Model file for the job. Use its own axes, mm. Face numbers are marked on the shaded views. A direction names the side the tool comes from. Round coordinates to 2 decimals unless told otherwise and drop trailing zeros. Order: outer loops, then holes, each group sorted by start corner. A loop starts at its lowest first (then second) coordinate and runs counter-clockwise, first axis right, second up. Notation, with made-up numbers: (51, -25) - (96, -25) arc R9 ccw to (96, -14) - close; hole circle Ø3 at (-3, -21.75). An arc over 180 degrees is marked (long way). Write item = value, one per line.
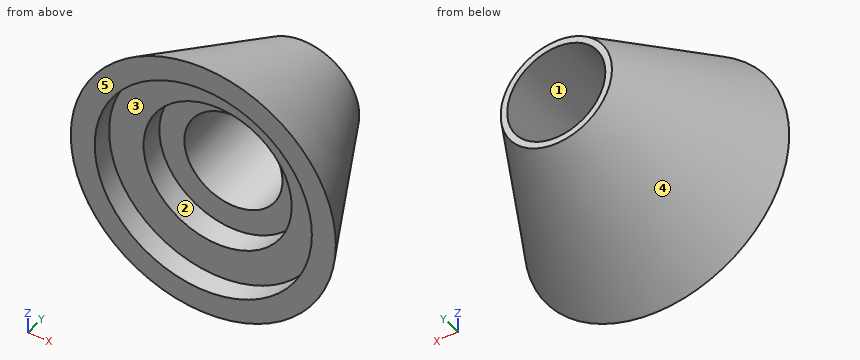
```python
from build123d import *

# Parameters (mm, degrees)
F2_R     = 4.702761
F3_DEPTH = 25.4
F5_R     = 7.100164
F6_DEPTH = 4.4196
F7_R     = 10.405199
F8_DEPTH = 2.1082


with BuildPart() as f1:
    # F0 (on Top) → F1 (revolve)
    with BuildSketch(Plane.XY):
        Polygon((0, -10.469328), (0, 4.262672), (-5.334, 4.262672), (-12.7, -10.469328), align=None)
    revolve(axis=Axis((0, 2.230672, 0), (0, -1, 0)))

    # F2 (on face) → F3 (cut)
    with BuildSketch(Plane(origin=(0, 4.262672, 0), x_dir=(-1, 0, 0), z_dir=(0, 1, 0))):
        Circle(F2_R)
    extrude(amount=-F3_DEPTH, mode=Mode.SUBTRACT)

    # F5 (on face) → F6 (cut)
    with BuildSketch(Plane.XZ.offset(10.469328)):
        Circle(F5_R)
    extrude(amount=-F6_DEPTH, mode=Mode.SUBTRACT)

    # F7 (on face) → F8 (cut)
    with BuildSketch(Plane.XZ.offset(10.469328)):
        Circle(F7_R)
    extrude(amount=-F8_DEPTH, mode=Mode.SUBTRACT)


solid = f1.part
```
1) Wall check: line 1 along X through (y, z) = (-2.75, -0.5); line 2 along Z through (x, y) = (0.75, -4); line 3 along Z through (x, y) = (0, -9.35). Give the ranges that are in metal, low to high.
Conclusion:
line_1 = -8.83 to -4.68, 4.68 to 8.83
line_2 = -9.44 to -4.64, 4.64 to 9.44
line_3 = -12.14 to -10.41, 10.41 to 12.14
2) Cut at B-B (x = 0). Write the cut outline in (y, z).
Conclusion:
outline = (-10.47, -12.7) - (4.26, -5.33) - (4.26, -4.7) - (-6.05, -4.7) - (-6.05, -7.1) - (-8.36, -7.1) - (-8.36, -10.41) - (-10.47, -10.41) - close; (-10.47, 10.41) - (-8.36, 10.41) - (-8.36, 7.1) - (-6.05, 7.1) - (-6.05, 4.7) - (4.26, 4.7) - (4.26, 5.33) - (-10.47, 12.7) - close
3) Cut at D-D (y = -1.5). Write the cut outline in (x, z), and give its area (3 significant figures).
Conclusion:
outline = circle Ø16.43 at (0, 0); hole circle Ø9.41 at (0, 0)
area = 143 mm^2
4) 3-axis set-ups, long thin cutter, end or side, ignore diameter. For the marked faces 1 and 2: which of +Z, -Z, +X, -X, +Y, -Y reach the whole face in a straight line?
Conclusion:
face_1 = +Y, -Y
face_2 = -Y
5) Mould opens along X. For the marked faces 3, 4 and 5 say: +X half, -X half, draft (parallel to the pull), parting line (faces both ways), or undercut.
Conclusion:
face_3 = undercut
face_4 = parting line
face_5 = draft
6) Cut at C-C (y = -7). Write the cut outline in (x, z), and give its area (3 significant figures).
Conclusion:
outline = circle Ø21.93 at (0, 0); hole circle Ø14.2 at (0, 0)
area = 219 mm^2
7) Flat gauge pins, fed straight in: pin 1 Ø5 at (y, z) = (1.5, -4.5) entering from +X; pin 2 Ø4 at (y, z) = (-3, -9.5) entering from -X; pin 3 Ø5 at (y, z) = (-1.5, 9.5) entering from +X. Where does each tip first touch, or does it go through?
Conclusion:
pin_1 = 7.11
pin_2 = -5.41
pin_3 = 4.94
8) Cut at A-A (z = 0). Write the cut outline in (x, y), and give its area (3 significant figures).
Conclusion:
outline = (-12.7, -10.47) - (-10.41, -10.47) - (-10.41, -8.36) - (-7.1, -8.36) - (-7.1, -6.05) - (-4.7, -6.05) - (-4.7, 4.26) - (-5.33, 4.26) - close; (4.7, -6.05) - (7.1, -6.05) - (7.1, -8.36) - (10.41, -8.36) - (10.41, -10.47) - (12.7, -10.47) - (5.33, 4.26) - (4.7, 4.26) - close
area = 92.0 mm^2
